Read the model definition and answer for the solid it produces. Units are mm, in the model's axes. Give positions to 0.01 mm unless a question says otherwise; leave off trailing zeros. Write each loop counter-clockwise with the first axis right and the second up, starting at its lowest first coordinate (ties: lowest second). Pieces come first, ordered by that corner, then holes. Notation, with made-up numbers: (-9.5, 54) -> (39.5, 54) arc R13 ccw to (39.5, 72) -> close; hole circle Ø10 at (23, -14). An arc over 180 degrees is marked (long way). Use a Markdown table: item, result.
from build123d import *

# Parameters (mm, degrees)
SKETCH1_W            = 254
SKETCH1_H            = 21.59
WALL_BASE_DEPTH      = 5.08
SKETCH2_W            = 25.4
SKETCH2_H            = 5.08
TAB_DEPTH            = 5.08
SKETCH7_W            = 25.4
SKETCH7_H            = 5.08
BOSS_EXTRUDE1_DEPTH  = 5.08
SKETCH3_RX           = 31.75
SKETCH3_RY           = 15.515530829
WHEEL_WELL_CUT_DEPTH = 129.089117512
SKETCH6_W            = 76.2
SKETCH6_H            = 5.461
CUT_EXTRUDE5_DEPTH   = 129.089117627
FILLET2_R            = 5.08


with BuildPart() as part:
    # Sketch1 → Wall-Base (new body)
    with BuildSketch(Plane(origin=(0, 0, 0), x_dir=(1, 0, 0), z_dir=(0, 1, 0))):
        Rectangle(SKETCH1_W, SKETCH1_H)
    extrude(amount=WALL_BASE_DEPTH)

    # Sketch2 → Tab (add)
    with BuildSketch(Plane(origin=(0, 0, -10.795), x_dir=(-1, 0, 0), z_dir=(0, 0, -1))):
        with Locations((38.1, 2.54)):
            Rectangle(SKETCH2_W, SKETCH2_H)
    tab = extrude(amount=TAB_DEPTH)

    # Sketch7 → Boss-Extrude1 (add)
    with BuildSketch(Plane.XY.offset(10.795)):
        with Locations((-72.39, 2.54)):
            Rectangle(SKETCH7_W, SKETCH7_H)
    boss_extrude1 = extrude(amount=BOSS_EXTRUDE1_DEPTH)

    # Mirror1: Tab across plane
    add(tab.mirror(Plane.ZY))

    # Sketch3 → Wheel-Well-Cut (cut, through all)
    with BuildSketch(Plane(origin=(0, 5.08, 0), x_dir=(1, 0, 0), z_dir=(0, 1, 0))):
        with Locations(Location((0, -10.795), (0, 0, 0))):
            Ellipse(SKETCH3_RX, SKETCH3_RY)
    extrude(amount=-WHEEL_WELL_CUT_DEPTH, mode=Mode.SUBTRACT)

    # Sketch6 → Cut-Extrude5 (cut, through all)
    with BuildSketch(Plane(origin=(0, 5.08, 0), x_dir=(1, 0, 0), z_dir=(0, 1, 0))):
        with Locations((-88.9, 5.5245)):
            Rectangle(SKETCH6_W, SKETCH6_H)
    cut_extrude5 = extrude(amount=-CUT_EXTRUDE5_DEPTH, mode=Mode.SUBTRACT)

    # Mirror4: Cut-Extrude5 across plane
    add(cut_extrude5.mirror(Plane.ZY), mode=Mode.SUBTRACT)

    # Fillet2
    # the kernel refuses this fillet: 5.08 mm, written as the material it takes off along each edge
    with BuildSketch(Plane(origin=(127, -12.7, 10.795), x_dir=(0, 0, -1), z_dir=(0, 1, 0)), Plane(origin=(-127, -12.7, 10.795), x_dir=(1, 0, 0), z_dir=(0, 1, 0))) as fillet2_piece_1:
        with BuildLine():
            CenterArc((FILLET2_R, FILLET2_R), FILLET2_R, 180, 90)
            Line((0, FILLET2_R), (-FILLET2_R * 0.02, FILLET2_R))
            Line((-FILLET2_R * 0.02, FILLET2_R), (-FILLET2_R * 0.02, -FILLET2_R * 0.02))
            Line((-FILLET2_R * 0.02, -FILLET2_R * 0.02), (FILLET2_R, -FILLET2_R * 0.02))
            Line((FILLET2_R, -FILLET2_R * 0.02), (FILLET2_R, 0))
        make_face()
    extrude(amount=30.48, mode=Mode.SUBTRACT)
    with BuildSketch(Plane(origin=(-127, -10.998522628, -10.795), x_dir=(0, 0, 1), z_dir=(0, 1, 0))) as fillet2_piece_2:
        with BuildLine():
            CenterArc((5.08, 4.399409051), FILLET2_R, 180, 60)
            Line((0, 4.399409051), (-0.1016, 4.399409051))
            Line((-0.1016, 4.399409051), (-0.1016, 0))
            Line((-0.1016, 0), (0, -0.1016))
            ThreePointArc((0, -0.1016), (1.27, -0.1016), (2.4892, -0.087988181))
            Line((2.4892, -0.087988181), (2.54, 0))
        make_face()
    extrude(amount=27.077045256, mode=Mode.SUBTRACT)
    with BuildSketch(Plane(origin=(127, -10.998522628, -10.795), x_dir=(-1, 0, 0), z_dir=(0, 1, 0))) as fillet2_piece_3:
        with BuildLine():
            CenterArc((4.399409051, 5.08), FILLET2_R, 210, 60)
            Line((0, 2.54), (-0.087988181, 2.4892))
            ThreePointArc((-0.087988181, 2.4892), (-0.1016, 1.27), (-0.1016, 0))
            Line((-0.1016, 0), (0, -0.1016))
            Line((0, -0.1016), (4.399409051, -0.1016))
            Line((4.399409051, -0.1016), (4.399409051, 0))
        make_face()
    extrude(amount=27.077045256, mode=Mode.SUBTRACT)

    # Mirror5: Boss-Extrude1 across plane
    add(boss_extrude1.mirror(Plane.ZY))


solid = part.part
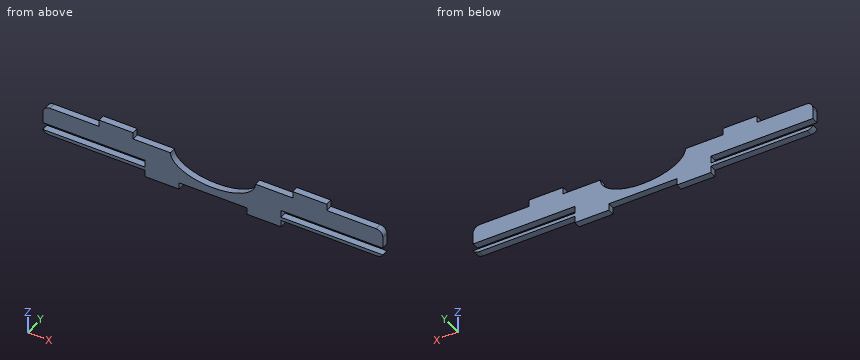
Item 1: Straight lines are drawn through the part: line 1 along Z through (x, y) = (-112.5, 1.6) (3 decimals); line 2 along X through (y, z) = (1.6, -12); line 3 along Z through (x, y) = (-77, 0.7) (3 decimals). For each, find the intervals that lie inside material, in ascending order. Write a range as [from, to].
Return value:
| item | result |
|---|---|
| line 1 | [-10.795, -8.255], [-2.794, 10.795] |
| line 2 | [-50.8, -25.4], [25.4, 50.8] |
| line 3 | [-10.795, -8.255], [-2.794, 15.875] |
Item 2: A cutting plane is placed at A-A (x = -62). Give the vertices of the cut face in (y, z) (3 decimals), then the cut area to 3 significant figures.
Return value:
| item | result |
|---|---|
| outline | (0, -10.795) -> (5.08, -10.795) -> (5.08, -8.255) -> (0, -8.255) -> close; (0, -2.794) -> (5.08, -2.794) -> (5.08, 15.875) -> (0, 15.875) -> close |
| area | 108 mm^2 |
Item 3: Each of these flat-tipped pins is pushed along its axis until it touches: P1, Ø2.5, axis at x = 101.5, y = 3, coming from the -Z side (3 decimals); P2, Ø2.5, axis at y = 3.5, z = -6, coming from the -X side; P3, Ø1.5, axis at x = -87, y = 3, coming from the +Z side (3 decimals). Where does it stop, or does it pass through?
Return value:
| item | result |
|---|---|
| P1 | z = -10.795 |
| P2 | x = -50.8 |
| P3 | z = 10.795 |
Item 4: A cutting plane is placed at B-B (x = 106). Give the vertices of the cut face in (y, z) (3 decimals).
Return value:
| item | result |
|---|---|
| outline | (0, -10.795) -> (5.08, -10.795) -> (5.08, -8.255) -> (0, -8.255) -> close; (0, -2.794) -> (5.08, -2.794) -> (5.08, 10.795) -> (0, 10.795) -> close |
